For this review, use the dimensioned drawing (mm, ordinates from the lowest corner) and the shaded views. A direction names the side the tool comes from. Give positions to 0.01 mm unless a question says otherwise; leave off trailing zeros. Write each loop counter-clockwise with the first axis right and the second up, starting at its lowest first coordinate (ties: lowest second). Pieces come first, ordered by that corner, then holes. Notation, with made-up numbers: M 29.25,-5 L 67.25,-5 A27 cw 67.25,33 Z; hole C -6,3 d9. An arc over 180 degrees is marked long. One line per item, written item: value. Start each with the question number.
Item 1: Tool access review of the marked faces 4 and 5: name each direction out of +Z, -Z, +X, -X, +Y, -Y from which nothing blocks a thin tool from reaching the whole face with its end or side.
Item 2: Mouldability with a two-part tool opening along X and no side actions: class the marked faces 1, 2 and 3 as released by +X, released by -X, zero draft, split by the parting line, or undercut.
Item 3: Clearance check with a flat-ended pin moving along its axis: pin 1 Ø1 at (x, z) = (140.5, 63.5) entering from +Y. State where the tip first meets the part, or that it passes through.
Item 4: Consider section A-A, the plane z = 46. Write out the cut boundary in (x, y).
Item 5: Consider section B-B, the plane x = 79. Write out the cut boundary in (y, z), and give its area (3 significant figures).
Item 6: To check wall thickness, follow probe 1 along X at (y, z) = (12.5, 56); probe 2 along X at (y, z) = (2.5, 46); probe 3 along Z at (x, y) = (67, 11). State the ranges of each line that lie inside material, in increasing order.
Item 7: Consider section D-D, the plane x = 128.5. Write out the cut boundary in (y, z), and give its area (3 significant figures).
Item 8: Consider section C-C, the plane y = 21.25. Write out the cut boundary in (x, z), and give its area (3 significant figures).
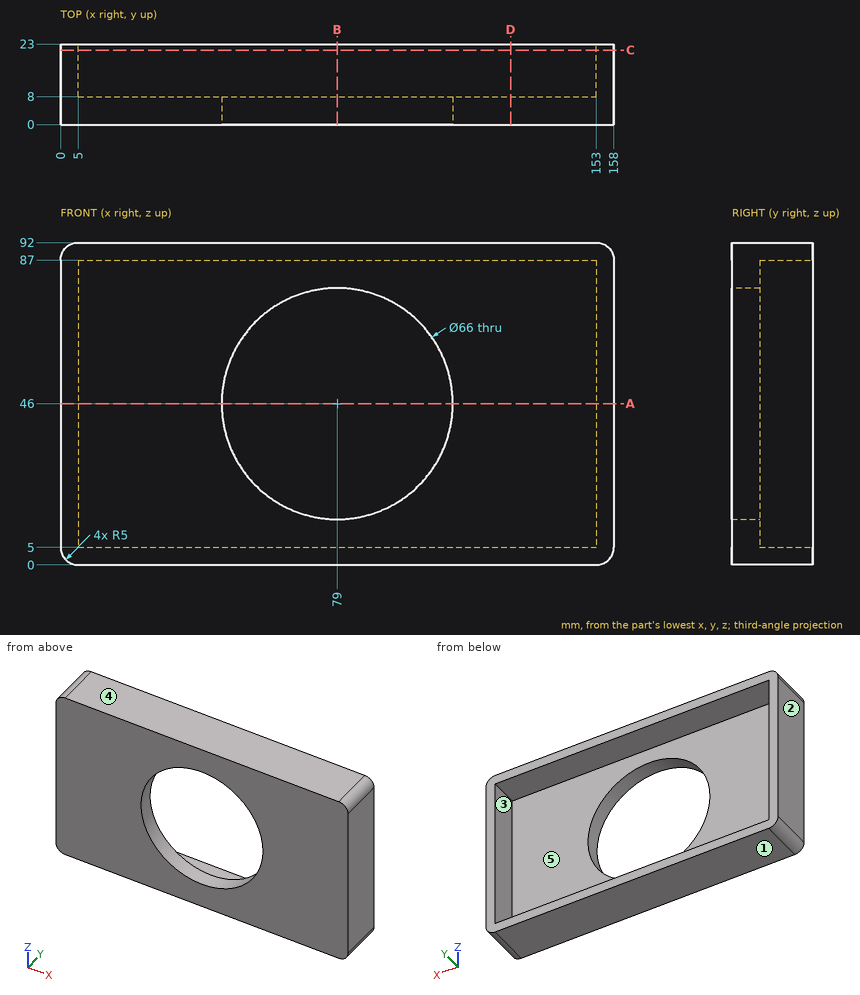
Model answer:
1. face 4: +Z, +X, -X, +Y, -Y
1. face 5: +Y
2. face 1: zero draft
2. face 2: released by -X
2. face 3: undercut
3. pin 1: stops at y = 8
4. outline: M 0,0 L 46,0 L 46,8 L 5,8 L 5,23 L 0,23 Z; M 112,0 L 158,0 L 158,23 L 153,23 L 153,8 L 112,8 Z
5. outline: M 0,0 L 23,0 L 23,5 L 8,5 L 8,13 L 0,13 Z; M 0,79 L 8,79 L 8,87 L 23,87 L 23,92 L 0,92 Z
5. area: 358 mm2
6. probe 1: x = 0 to 5, 153 to 158
6. probe 2: x = 0 to 46, 112 to 158
6. probe 3: z = 0 to 5, 87 to 92
7. outline: M 0,0 L 23,0 L 23,5 L 8,5 L 8,87 L 23,87 L 23,92 L 0,92 Z
7. area: 886 mm2
8. outline: M 0,5 A5 ccw 5,0 L 153,0 A5 ccw 158,5 L 158,87 A5 ccw 153,92 L 5,92 A5 ccw 0,87 Z; hole M 5,5 L 153,5 L 153,87 L 5,87 Z
8. area: 2,380 mm2
